Could you check a few things on this model? Use its own coordinates, in mm. A direction names the side the tool comes from. Round coordinates to 2 decimals unless told otherwise and drop trailing zeros. Loops run counter-clockwise (first coordinate to the right, second up) from the corner with the lowest first, then second, coordinate; pieces in that order, holes last. Notation, with made-up numbers: M 73.5,38 L 107.5,38 A14 cw 107.5,61 Z; hole C 63.25,3 d6. An arc over 180 degrees is marked long. Answer in a Markdown table with one row per item.
```python
from build123d import *

# Parameters (mm, degrees)
DODANIE_WYCI_GNI_CIE1_DEPTH      = 27.5
DODANIE_WYCI_GNI_CIE1_DEPTH_BACK = 27.5
SZKIC1_R                         = 8
WYTNIJ_WYCI_GNI_CIE3_DEPTH       = 262.225344217
WYTNIJ_WYCI_GNI_CIE3_DEPTH_BACK  = 262.225344217
SZKIC2_W                         = 50
SZKIC2_H                         = 271.010465283
DODANIE_WYCI_GNI_CIE2_DEPTH      = 32.5
DODANIE_WYCI_GNI_CIE2_DEPTH_BACK = 32.5
SZKIC4_R                         = 5
WYTNIJ_WYCI_GNI_CIE4_DEPTH       = 262.79893136
WYTNIJ_WYCI_GNI_CIE4_DEPTH_BACK  = 262.79893136
SZKIC5_W                         = 50
SZKIC5_H                         = 2
SZKIC7_R                         = 8
WYTNIJ_WYCI_GNI_CIE5_DEPTH       = 267.612885025
ZAOKR_GLENIE1_R                  = 5


with BuildPart() as part:
    # Szkic1 → Dodanie-wyciągnięcie1 (new, two sides: drawn at the far end of the back side and taken through both)
    with BuildSketch(Plane(origin=(0, 0, 0), x_dir=(0, 0, -1), z_dir=(1, 0, 0)).offset(-DODANIE_WYCI_GNI_CIE1_DEPTH_BACK)):
        with BuildLine():
            Line((20, 0), (20, 26.995226764))
            ThreePointArc((20, 26.995226764), (14.862367943, 101.995226764), (20, 176.995226764))
            ThreePointArc((20, 176.995226764), (21.196911631, 202.008236386), (19.543563623, 226.995226764))
            ThreePointArc((19.543563623, 226.995226764), (-10.032375571, 253.010105435), (-39.350561597, 226.705085769))
            Line((-39.350561597, 226.705085769), (-45, 176.995226764))
            ThreePointArc((-45, 176.995226764), (-48.517838539, 114.888486347), (-45, 52.781745931))
            Line((-45, 52.781745931), (-58.890872965, 38.890872965))
            Line((-58.890872965, 38.890872965), (-20, 0))
            ThreePointArc((-20, 0), (0, -20), (20, 0))
        make_face()
        Circle(SZKIC1_R, mode=Mode.SUBTRACT)
    extrude(amount=DODANIE_WYCI_GNI_CIE1_DEPTH + DODANIE_WYCI_GNI_CIE1_DEPTH_BACK)

    # Szkic2 → Wytnij-wyciągnięcie3 (cut, two sides: drawn at the far end of the back side and taken through both)
    with BuildSketch(Plane.XY.offset(-WYTNIJ_WYCI_GNI_CIE3_DEPTH_BACK)):
        with Locations((0, 115.505232642)):
            Rectangle(SZKIC2_W, SZKIC2_H)
    extrude(amount=WYTNIJ_WYCI_GNI_CIE3_DEPTH + WYTNIJ_WYCI_GNI_CIE3_DEPTH_BACK, mode=Mode.SUBTRACT)

    # Szkic4 → Dodanie-wyciągnięcie2 (add, two sides: drawn at the far end of the back side and taken through both)
    with BuildSketch(Plane(origin=(0, 0, 0), x_dir=(0, 0, -1), z_dir=(1, 0, 0)).offset(-DODANIE_WYCI_GNI_CIE2_DEPTH_BACK)):
        with Locations((12, 26.995226764)):
            Circle(SZKIC4_R)
        with Locations((0, 101.995226764)):
            Circle(SZKIC4_R)
        with Locations((12, 176.995226764)):
            Circle(SZKIC4_R)
        with Locations((-36.948502055, 176.995226764)):
            Circle(SZKIC4_R)
        with Locations((-9.886287655, 223.356522646)):
            Circle(SZKIC4_R)
    extrude(amount=DODANIE_WYCI_GNI_CIE2_DEPTH + DODANIE_WYCI_GNI_CIE2_DEPTH_BACK)

    # Szkic5 → Wytnij-wyciągnięcie4 (cut, two sides: drawn at the far end of the back side and taken through both)
    with BuildSketch(Plane.XY.offset(-WYTNIJ_WYCI_GNI_CIE4_DEPTH_BACK)):
        with Locations((0, 252.010465283)):
            Rectangle(SZKIC5_W, SZKIC5_H)
    extrude(amount=WYTNIJ_WYCI_GNI_CIE4_DEPTH + WYTNIJ_WYCI_GNI_CIE4_DEPTH_BACK, mode=Mode.SUBTRACT)

    # Szkic7 → Wytnij-wyciągnięcie5 (cut, through all)
    with BuildSketch(Plane(origin=(27.5, 0, 0), x_dir=(0, 0, -1), z_dir=(1, 0, 0))):
        with Locations((-10.032375571, 200)):
            Circle(SZKIC7_R)
        with Locations((-10.032375571, 160)):
            Circle(SZKIC7_R)
        with Locations((-10.032375571, 120)):
            Circle(SZKIC7_R)
        with BuildLine():
            ThreePointArc((-42.868867151, 160.416733268), (-44.454199067, 133.445260635), (-44.703970192, 106.428391318))
            ThreePointArc((-44.703970192, 106.428391318), (-39.627132181, 101.506428721), (-34.705169584, 106.583266732))
            ThreePointArc((-34.705169584, 106.583266732), (-34.459970914, 133.105549545), (-32.903661004, 159.583266732))
            ThreePointArc((-32.903661004, 159.583266732), (-37.46953081, 164.982603073), (-42.868867151, 160.416733268))
        make_face()
        with BuildLine():
            ThreePointArc((-4.998947211, 90.299199015), (-4.066241956, 67.369334541), (-2.211268005, 44.495600794))
            ThreePointArc((-2.211268005, 44.495600794), (3.267624284, 40.025506916), (7.737718162, 45.504399206))
            ThreePointArc((7.737718162, 45.504399206), (5.91528868, 67.976826233), (4.998947211, 90.504399206))
            ThreePointArc((4.998947211, 90.504399206), (-0.102600095, 95.400746322), (-4.998947211, 90.299199015))
        make_face()
    extrude(amount=-WYTNIJ_WYCI_GNI_CIE5_DEPTH, mode=Mode.SUBTRACT)

    # Zaokrąglenie1
    zaokr_glenie1_edges = [part.edges().sort_by_distance(p)[0] for p in [
        (-26.25, 0, 20),
        (-26.25, 38.890872965, 58.890872965),
        (-26.25, 52.781745931, 45),
        (-26.25, 26.995226764, -20),
        (26.25, 26.995226764, -20),
        (26.25, 52.781745931, 45),
        (26.25, 38.890872965, 58.890872965),
        (26.25, 0, 20),
    ]]
    fillet(zaokr_glenie1_edges, radius=ZAOKR_GLENIE1_R)


solid = part.part
```
1) I need wall thicknesses on line 1 (X direction, y = 206.5, z = 2); line 2 (Y direction, x = 26, z = 0); line 3 (Y direction, x = 2, z = -12). Which ranges of each line are inside material? Lowest first, please.
Computed:
| item | result |
|---|---|
| line 1 | x = -27.5 to -25, 25 to 27.5 |
| line 2 | y = -20 to -8, 8 to 40.83, 95.4 to 251.31 |
| line 3 | y = 22 to 32, 172 to 182 |
2) I want a section at C-C, the plane z = 27.5. Please give me the cut outline in (x, y).
Computed:
| item | result |
|---|---|
| outline | M -27.5,7.5 L -25,7.5 L -25,247.21 L -27.5,247.21 Z; M 25,7.5 L 27.5,7.5 L 27.5,247.21 L 25,247.21 Z |
3) If we mould it in two halves opening along Y, with no side actions, what happens to faces 6 (the face through (-30.04, 172.56, 34.64)), 7 (the face through (26.3, 95.4, 0)), 8 (the face through (-32.5, 223, 10))? For each: released by +Y, released by -Y, zero draft, split by the parting line, or undercut.
Computed:
| item | result |
|---|---|
| face 6 | split by the parting line |
| face 7 | undercut |
| face 8 | zero draft |
4) Which directions (+Z, -Z, +X, -X, +Y, -Y) give clear straight access to the entire face, cutting with the end or side of a thin tool? Please do faces 1 (the face through (-30.035, 228.314, 10.537)), 2 (the face through (26.268, 164.972, 37.36)), 3 (the face through (29.97, 172.56, 34.64)), 4 (the face through (-0.35, 106.21, -2.69)), 5 (the face through (26.232, 253.007, 9.429)).
Computed:
| item | result |
|---|---|
| face 1 | -X |
| face 2 | +X, -X |
| face 3 | +X |
| face 4 | none |
| face 5 | +X, -X, +Y |
5) Will these pins go through, and if not, where does the flat tip stop? P1, Ø6, axis at x = -23.5, z = 44.5, coming from the -Y side; P2, Ø10, axis at x = -17, z = 3, coming from the -Y side; P3, Ø2, axis at y = 35.5, z = 38.5, coming from the -X side.
Computed:
| item | result |
|---|---|
| P1 | stops at y = 21.9 |
| P2 | stops at y = 97 |
| P3 | stops at x = -27.5 |
6) I want a section at D-D, the plane x = -15.5. Please give me the cut outline in (y, z).
Computed:
| item | result |
|---|---|
| outline | C 27,-12 d10; C 102,0 d10; C 177,-12 d10; C 177,36.95 d10; C 223.36,9.89 d10 |
7) I want a section at B-B, the plane y = 120. Please give me the cut outline in (x, z).
Computed:
| item | result |
|---|---|
| outline | M -27.5,-15.16 L -25,-15.16 L -25,2.03 L -27.5,2.03 Z; M -27.5,18.03 L -25,18.03 L -25,34.75 L -27.5,34.75 Z; M -27.5,44.75 L -25,44.75 L -25,48.49 L -27.5,48.49 Z; M 25,-15.16 L 27.5,-15.16 L 27.5,2.03 L 25,2.03 Z; M 25,18.03 L 27.5,18.03 L 27.5,34.75 L 25,34.75 Z; M 25,44.75 L 27.5,44.75 L 27.5,48.49 L 25,48.49 Z |
8) I want a section at A-A, the plane y = 62.5. Please give me the cut outline in (x, z).
Computed:
| item | result |
|---|---|
| outline | M -27.5,-16.28 L -25,-16.28 L -25,-6.28 L -27.5,-6.28 Z; M -27.5,3.75 L -25,3.75 L -25,46.02 L -27.5,46.02 Z; M 25,-16.28 L 27.5,-16.28 L 27.5,-6.28 L 25,-6.28 Z; M 25,3.75 L 27.5,3.75 L 27.5,46.02 L 25,46.02 Z |
